```python
from build123d import *

# Parameters (mm, degrees)
BOSS_EXTRUDE1_DEPTH = 3.175
BOSS_EXTRUDE3_DEPTH = 3.175


with BuildPart() as part:
    # Sketch2 → Boss-Extrude1 (new body)
    with BuildSketch(Plane(origin=(0, 0, 0), x_dir=(1, 0, 0), z_dir=(0, 1, 0))):
        Polygon((3.2004, -6.35), (138.79195, -6.35), (138.79195, -3.175), (141.99235, -3.175), (141.99235, 0), (0, 0), (0, -3.175), (3.2004, -3.175), align=None)
    extrude(amount=BOSS_EXTRUDE1_DEPTH)

    # Sketch4 → Boss-Extrude3 (add)
    with BuildSketch(Plane(origin=(0, 3.175, 0), x_dir=(1, 0, 0), z_dir=(0, 1, 0))):
        Polygon((142.09395, -3.2766), (142.09395, 0.1016), (-0.1016, 0.1016), (-0.1016, -3.2766), (3.0988, -3.2766), (3.0988, -6.4516), (138.89355, -6.4516), (138.89355, -3.2766), align=None)
    extrude(amount=-BOSS_EXTRUDE3_DEPTH)


solid = part.part
```
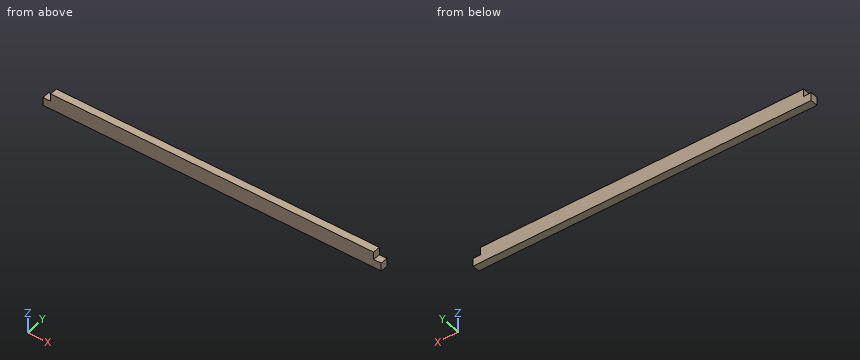
Design review of the part built by this model. Coordinates are the model's own, in mm. Coordinates: 2 decimals unless noted, no trailing zeros. Order: outer loops, then holes, each group sorted by start corner. A loop starts at its lowest first (then second) coordinate and runs counter-clockwise, first axis right, second up.
1) Wall thickness on line 1 along X through (y, z) = (2.45, 4): over which ranges is the line inside the solid? List them lowest first.
2) Take a section at B-B, the plane z = 4.5. Give the boundary of the cut face in (x, y) (3 decimals), and give its area (3 significant figures).
3) Take a section at A-A, the plane y = 2.6. Give the boundary of the cut face in (x, z), and give its area (3 significant figures).
4) Clearance check with flat-ended pins moving along their axes: pin 1 (1 mm diameter, centred on y = 1.5, z = 5.5, fed in from -X); pin 2 (1 mm diameter, centred on x = 1, y = 1, fed in from +Z); pin 3 (1.6 mm diameter, centred on y = 2, z = 5, fed in from +X). State where each tip first meets the part, or that it passes through.
Returned:
1. line 1: x = 3.1 to 138.89
2. outline: (3.099, 0) - (138.894, 0) - (138.894, 3.175) - (3.099, 3.175) - close
2. area: 431 mm2
3. outline: (-0.1, -0.1) - (142.09, -0.1) - (142.09, 3.28) - (138.89, 3.28) - (138.89, 6.45) - (3.1, 6.45) - (3.1, 3.28) - (-0.1, 3.28) - close
3. area: 912 mm2
4. pin 1: stops at x = 3.1
4. pin 2: stops at z = 3.28
4. pin 3: stops at x = 138.89
